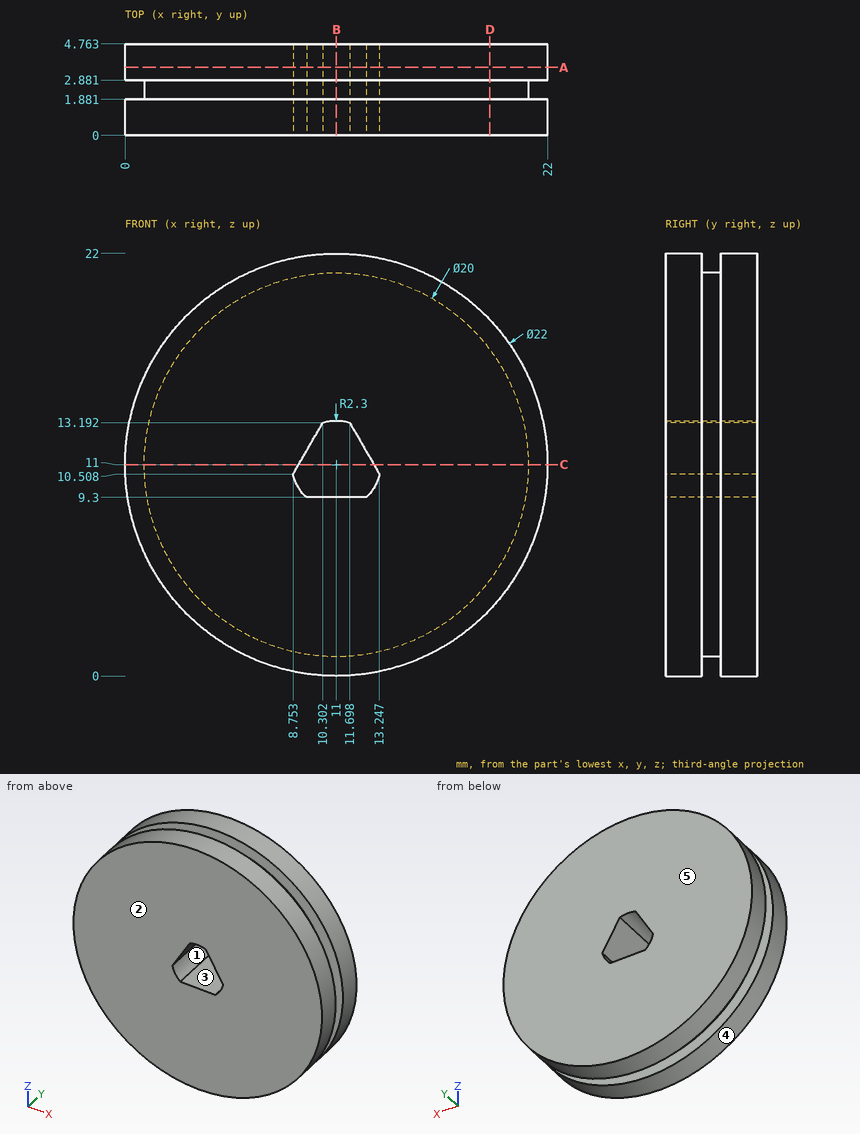
Could you check a few things on this drawing? It's one solid part, dimensions in mm from its lowest x, y, z. A direction names the side the tool comes from. Give positions to 0.01 mm unless a question says otherwise; leave off trailing zeros. Order: outer loops, then holes, each group sorted by start corner. A loop starts at its lowest first (then second) coordinate and runs counter-clockwise, first axis right, second up. Notation, with made-up numbers: (-5.5, 14.5) - (12.5, 14.5) arc R31 ccw to (12.5, 41.5) - close; hole circle Ø7 at (87, -13). An arc over 180 degrees is marked (long way). One line per item, written item: value. Start each with the question number.
1. If I drill on probe 1 along X at (y, z) = (4.4, 12) (1 decimal); probe 2 along Z at (x, y) = (11.25, 2.55); probe 3 along Z at (x, y) = (12.5, 0.5) (1 decimal), over which ranges is the centre line in solid material (lowest first)?
2. Imagine slicing it at C-C on z = 11. List the corners of the cut face in (x, y) for me.
3. Imagine slicing it at D-D on x = 19. List the corners of the cut face in (y, z) for me.
4. Imagine slicing it at A-A on y = 3.55. List the corners of the cut face in (x, z) for me, plus the area to 3 significant figures.
5. Imagine slicing it at B-B on x = 11. List the corners of the cut face in (y, z) for me.
6. Thinking about a two-plate mould opening in X: for the marked faces 3, 4 and 5, which applies, +X half, -X half, draft (parallel to the pull), parting line (faces both ways), or undercut?
7. For P1, Ø1.5, axis at x = 4, y = 4, coming from the -Z side; P2, Ø1.5, axis at y = 2, z = 16.5, coming from the -X side, each with a flat end and sliding along its axis, tell me the tip position at first contact or that it passes through.
8. For the marked faces 1 and 2, which set-ups out of +Z, -Z, +X, -X, +Y, -Y let a thin tool reach every point of the face, with its end or its side?
Values:
1. probe 1: 0 to 9.6, 12.4 to 22
1. probe 2: 1 to 9.3, 13.29 to 21
1. probe 3: 0.1 to 9.3, 11.8 to 21.9
2. outline: (0, 0) - (9.04, 0) - (9.04, 4.76) - (0, 4.76) - (0, 2.88) - (1, 2.88) - (1, 1.88) - (0, 1.88) - close; (12.96, 0) - (22, 0) - (22, 1.88) - (21, 1.88) - (21, 2.88) - (22, 2.88) - (22, 4.76) - (12.96, 4.76) - close
3. outline: (0, 3.45) - (1.88, 3.45) - (1.88, 5) - (2.88, 5) - (2.88, 3.45) - (4.76, 3.45) - (4.76, 18.55) - (2.88, 18.55) - (2.88, 17) - (1.88, 17) - (1.88, 18.55) - (0, 18.55) - close
4. outline: circle Ø22 at (11, 11); hole (8.75, 10.51) arc R2.3 ccw to (9.45, 9.3) - (12.55, 9.3) arc R2.3 ccw to (13.25, 10.51) - (11.7, 13.19) arc R2.3 ccw to (10.3, 13.19) - close
4. area: 367 mm²
5. outline: (0, 0) - (1.88, 0) - (1.88, 1) - (2.88, 1) - (2.88, 0) - (4.76, 0) - (4.76, 9.3) - (0, 9.3) - close; (0, 13.3) - (4.76, 13.3) - (4.76, 22) - (2.88, 22) - (2.88, 21) - (1.88, 21) - (1.88, 22) - (0, 22) - close
6. face 3: undercut
6. face 4: parting line
6. face 5: draft
7. P1: z = 1.95
7. P2: x = 1.08
8. face 1: +Y, -Y
8. face 2: +Z, -Z, +X, -X, -Y
